Build history of the part. All positions in model axes, mm. Face numbers are marked on the shaded views. Give positions to 0.01 mm unless a question says otherwise; leave off trailing zeros. Order: outer loops, then holes, each group sorted by start corner. A loop starts at its lowest first (then second) coordinate and runs counter-clockwise, first axis right, second up. Notation, with made-up numbers: (-32, 26) - (23, 26) arc R18 ccw to (23, 59) - close; hole circle Ø5 at (-22, -17.75). An arc over 180 degrees is marked (long way). Write each question's results on one line, items separated by ' | '. Start each with the question number.
1) Drill centre lines: line 1 along X through (y, z) = (56.35, 55); line 2 along X through (y, z) = (57.35, 55); line 3 along X through (y, z) = (53.25, 73). Where is each one in solid material? Low to high. Write a range as from..to.
2) Cut at C-C on y = 53. List the corners of the cut face in (x, z), plus the area to 3 significant figures.
3) Cut at A-A on z = 70. State how many separate pieces and enclosed holes the cut face has, plus the area to 3 significant figures.
4) Cut at B-B on z = 21. List the corners of the cut face in (x, y), plus the area to 3 significant figures.
5) Two-plate mould, pull along X, no slides. Class the marked faces 1, 2 and 3: +X half, -X half, draft (parallel to the pull), parting line (faces both ways), or undercut.
6) Cut at D-D on x = 18. List the corners of the cut face in (y, z), plus the area to 3 significant figures.
7) Drop flat-ended pins along their axis: pin 1 Ø3 at (x, z) = (13.89, 70) entering from +Y; pin 2 Ø1.1 at (y, z) = (57, 76) entering from -X; pin 3 Ø5 at (x, z) = (9, 66) entering from -Y; pin 4 Ø1.6 at (x, z) = (-1.11, 70) entering from -Y. Give the stop position or say it passes through.
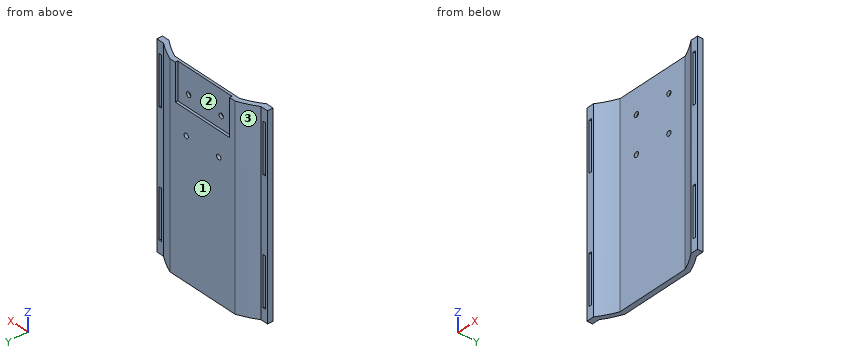
from build123d import *

# Parameters (mm, degrees)
BOSS_EXTRUDE1_DEPTH = 80
SKETCH8_W           = 25
SKETCH8_H           = 15
CUT_EXTRUDE2_DEPTH  = 1
SKETCH9_R           = 1
CUT_EXTRUDE3_DEPTH  = 1
SKETCH12_W          = 1
SKETCH12_H          = 20
CUT_EXTRUDE4_DEPTH  = 4.69
SKETCH13_R          = 1
CUT_EXTRUDE5_DEPTH  = 4.69


with BuildPart() as part:
    # Sketch4 → Boss-Extrude1 (new body)
    with BuildSketch(Plane.XY):
        with BuildLine():
            Line((-19.110677356, 53.885203774), (-16.110677356, 53.885203774))
            ThreePointArc((-16.110677356, 53.885203774), (-12.467042329, 56.084638099), (-8.610677356, 57.885203774))
            Line((-8.610677356, 57.885203774), (21.389322644, 57.885203774))
            ThreePointArc((21.389322644, 57.885203774), (25.245687617, 56.084638099), (28.889322644, 53.885203774))
            Line((28.889322644, 53.885203774), (31.889322644, 53.885203774))
            Line((31.889322644, 53.885203774), (31.889322644, 51.627366583))
            Line((31.889322644, 51.627366583), (28.889322644, 51.627366583))
            ThreePointArc((28.889322644, 51.627366583), (25.259796787, 53.968495283), (21.389322644, 55.885203774))
            Line((21.389322644, 55.885203774), (-8.610677356, 55.885203774))
            ThreePointArc((-8.610677356, 55.885203774), (-12.481151499, 53.968495283), (-16.110677356, 51.627366583))
            Line((-16.110677356, 51.627366583), (-19.110677356, 51.627366583))
            Line((-19.110677356, 51.627366583), (-19.110677356, 53.885203774))
        make_face()
    extrude(amount=BOSS_EXTRUDE1_DEPTH)

    # Sketch8 → Cut-Extrude2 (cut)
    with BuildSketch(Plane(origin=(0, 57.885203774, 0), x_dir=(1, 0, 0), z_dir=(0, 1, 0))):
        with Locations((6.389322644, -72.5)):
            Rectangle(SKETCH8_W, SKETCH8_H)
    extrude(amount=-CUT_EXTRUDE2_DEPTH, mode=Mode.SUBTRACT)

    # Sketch9 → Cut-Extrude3 (cut)
    with BuildSketch(Plane(origin=(0, 56.885203774, 0), x_dir=(1, 0, 0), z_dir=(0, 1, 0))):
        with Locations(Location((-1.110677356, -70, 0), (0, 0, 270))):
            Circle(SKETCH9_R)
        with Locations(Location((13.889322644, -70, 0), (0, 0, 270))):
            Circle(SKETCH9_R)
    extrude(amount=-CUT_EXTRUDE3_DEPTH, mode=Mode.SUBTRACT)

    # Sketch12 → Cut-Extrude4 (cut)
    with BuildSketch(Plane(origin=(0, 53.885203774, 0), x_dir=(1, 0, 0), z_dir=(0, 1, 0))):
        with Locations((-17.610677356, -15)):
            Rectangle(SKETCH12_W, SKETCH12_H)
        with Locations((-17.610677356, -65)):
            Rectangle(SKETCH12_W, SKETCH12_H)
        with Locations((30.389322644, -15)):
            Rectangle(SKETCH12_W, SKETCH12_H)
        with Locations((30.389322644, -65)):
            Rectangle(SKETCH12_W, SKETCH12_H)
    extrude(amount=-CUT_EXTRUDE4_DEPTH, mode=Mode.SUBTRACT)

    # Sketch13 → Cut-Extrude5 (cut)
    with BuildSketch(Plane(origin=(0, 57.885203774, 0), x_dir=(1, 0, 0), z_dir=(0, 1, 0))):
        with Locations(Location((-1.110677356, -55, 0), (0, 0, 270))):
            Circle(SKETCH13_R)
        with Locations(Location((13.889322644, -55, 0), (0, 0, 270))):
            Circle(SKETCH13_R)
    extrude(amount=-CUT_EXTRUDE5_DEPTH, mode=Mode.SUBTRACT)


solid = part.part
Results:
1) line 1: -11.96..-2.11, -0.11..12.89, 14.89..24.74 | line 2: -9.87..-2.11, -0.11..12.89, 14.89..22.65 | line 3: -19.11..-18.11, -17.11..-13.69, 26.47..29.89, 30.89..31.89
2) outline: (-19.11, 0) - (-14.09, 0) - (-14.09, 80) - (-19.11, 80) - close; (26.87, 0) - (31.89, 0) - (31.89, 80) - (26.87, 80) - close; hole (-18.11, 5) - (-17.11, 5) - (-17.11, 25) - (-18.11, 25) - close; hole (-18.11, 55) - (-17.11, 55) - (-17.11, 75) - (-18.11, 75) - close; hole (29.89, 5) - (30.89, 5) - (30.89, 25) - (29.89, 25) - close; hole (29.89, 55) - (30.89, 55) - (30.89, 75) - (29.89, 75) - close | area: 723 mm^2
3) separate pieces: 5 | enclosed holes: 0 | area: 71.7 mm^2
4) outline: (-19.11, 51.63) - (-18.11, 51.63) - (-18.11, 53.89) - (-19.11, 53.89) - close; (-17.11, 51.63) - (-16.11, 51.63) arc R38.22 cw to (-8.61, 55.89) - (21.39, 55.89) arc R38.22 cw to (28.89, 51.63) - (29.89, 51.63) - (29.89, 53.89) - (28.89, 53.89) arc R40.07 ccw to (21.39, 57.89) - (-8.61, 57.89) arc R40.07 ccw to (-16.11, 53.89) - (-17.11, 53.89) - close; (30.89, 51.63) - (31.89, 51.63) - (31.89, 53.89) - (30.89, 53.89) - close | area: 101 mm^2
5) face 1: draft | face 2: undercut | face 3: -X half
6) outline: (55.89, 0) - (57.89, 0) - (57.89, 65) - (56.89, 65) - (56.89, 80) - (55.89, 80) - close | area: 145 mm^2
7) pin 1: y = 56.89 | pin 2: x = -11.77 | pin 3: y = 55.89 | pin 4: through
